```python
from build123d import *

# Parameters (mm, degrees)
SKETCH_1_R          = 16.5
EXTRUDE_1_DEPTH     = 22.7
SKETCH_2_R          = 18.5
EXTRUDE_2_DEPTH     = 19
SKETCH_3_R          = 1.5
CUT_EXTRUDE_1_DEPTH = 2
SKETCH_4_R          = 5.5
EXTRUDE_3_DEPTH     = 6
SKETCH_5_R          = 3
EXTRUDE_4_DEPTH     = 15.5
SKETCH_6_R          = 5
EXTRUDE_5_DEPTH     = 2.8
SKETCH_7_W          = 3.619294394
SKETCH_7_H          = 1.78180647
EXTRUDE_6_DEPTH     = 3.5


with BuildPart() as part:
    # 草图1 → 凸台-拉伸1 (new body)
    with BuildSketch(Plane.XY):
        Circle(SKETCH_1_R)
    extrude(amount=EXTRUDE_1_DEPTH)

    # 草图2 → 凸台-拉伸2 (add)
    with BuildSketch(Plane.XY.offset(22.7)):
        Circle(SKETCH_2_R)
    extrude(amount=EXTRUDE_2_DEPTH)

    # 草图3 → 切除-拉伸1 (cut)
    with BuildSketch(Plane.XY.offset(41.7)):
        with Locations((15.5, 0)):
            Circle(SKETCH_3_R)
        with Locations((7.75, -13.423393759)):
            Circle(SKETCH_3_R)
        with Locations((-7.75, -13.423393759)):
            Circle(SKETCH_3_R)
        with Locations((-15.5, 0)):
            Circle(SKETCH_3_R)
        with Locations((-7.75, 13.423393759)):
            Circle(SKETCH_3_R)
        with Locations((7.75, 13.423393759)):
            Circle(SKETCH_3_R)
    extrude(amount=-CUT_EXTRUDE_1_DEPTH, mode=Mode.SUBTRACT)

    # 草图4 → 凸台-拉伸3 (add)
    with BuildSketch(Plane.XY.offset(41.7)):
        with Locations((0, 7)):
            Circle(SKETCH_4_R)
    extrude(amount=EXTRUDE_3_DEPTH)

    # 草图5 → 凸台-拉伸4 (add)
    with BuildSketch(Plane.XY.offset(47.7)):
        with Locations((0, 7)):
            Circle(SKETCH_5_R)
    extrude(amount=EXTRUDE_4_DEPTH)

    # 草图6 → 凸台-拉伸5 (add)
    with BuildSketch(Plane(origin=(0, 0, 0), x_dir=(-1, 0, 0), z_dir=(0, 0, -1))):
        Circle(SKETCH_6_R)
    extrude(amount=EXTRUDE_5_DEPTH)

    # 草图7 → 凸台-拉伸6 (add)
    with BuildSketch(Plane(origin=(0, 0, 0), x_dir=(-1, 0, 0), z_dir=(0, 0, -1))):
        with Locations((0, 11.99935295)):
            Rectangle(SKETCH_7_W, SKETCH_7_H)
        with Locations((0, -11.99935295)):
            Rectangle(SKETCH_7_W, SKETCH_7_H)
    extrude(amount=EXTRUDE_6_DEPTH)


solid = part.part
```
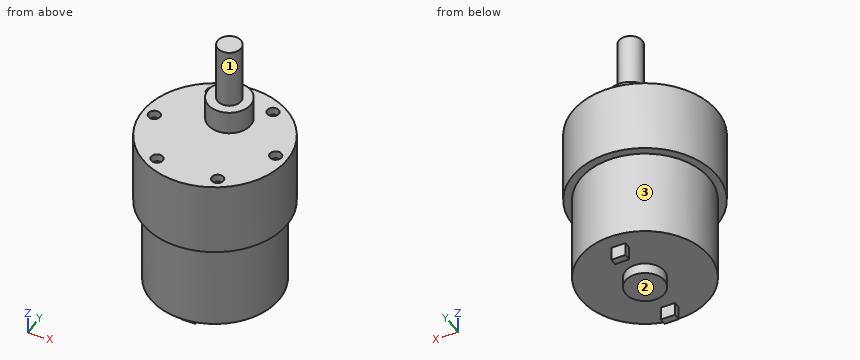
The model under review builds one solid part; all positions refer to its coordinate system, in mm. Face numbers are marked on the shaded views. A direction names the side the tool comes from. Round coordinates to 2 decimals unless told otherwise and drop trailing zeros. Order: outer loops, then holes, each group sorted by start corner. A loop starts at its lowest first (then second) coordinate and runs counter-clockwise, first axis right, second up. Notation, with made-up numbers: (40, -18.75) -> (87, -18.75) arc R13 ccw to (87, -3.75) -> close; hole circle Ø4 at (-9.5, 35.5). An arc over 180 degrees is marked (long way). Use a Markdown table: item, result.
Q1. For line 1 (Y direction, x = 7.75, z = 40.25); line 2 (Z direction, x = 13.5, y = 11); line 3 (Z direction, x = 15, y = 2.5), list the stretches that pass through material, from the lowest coordinate up.
Values:
| item | result |
|---|---|
| line 1 | y = -16.8 to -14.92, -11.92 to 11.92, 14.92 to 16.8 |
| line 2 | z = 22.7 to 41.7 |
| line 3 | z = 0 to 41.7 |
Q2. We need section B-B on x = 0. Write out the cut boundary in (y, z).
Values:
| item | result |
|---|---|
| outline | (-18.5, 22.7) -> (-16.5, 22.7) -> (-16.5, 0) -> (-12.89, 0) -> (-12.89, -3.5) -> (-11.11, -3.5) -> (-11.11, 0) -> (-5, 0) -> (-5, -2.8) -> (5, -2.8) -> (5, 0) -> (11.11, 0) -> (11.11, -3.5) -> (12.89, -3.5) -> (12.89, 0) -> (16.5, 0) -> (16.5, 22.7) -> (18.5, 22.7) -> (18.5, 41.7) -> (12.5, 41.7) -> (12.5, 47.7) -> (10, 47.7) -> (10, 63.2) -> (4, 63.2) -> (4, 47.7) -> (1.5, 47.7) -> (1.5, 41.7) -> (-18.5, 41.7) -> close |
Q3. Tool access review of the marked faces 1, 2 and 3: name each direction out of +Z, -Z, +X, -X, +Y, -Y from which nothing blocks a thin tool from reaching the whole face with its end or side.
Values:
| item | result |
|---|---|
| face 1 | +Z |
| face 2 | -Z, +X, -X |
| face 3 | -Z |
Q4. Clearance check with flat-ended pins moving along their axes: P1, Ø1.4, axis at y = -12, z = -1.5, coming from the -X side; P2, Ø6, axis at x = 0, y = 14, coming from the +Z side; P3, Ø2.5, axis at x = -15.5, y = -0.5, coming from the +Z side. State where each tip first meets the part, or that it passes through.
Values:
| item | result |
|---|---|
| P1 | stops at x = -1.81 |
| P2 | stops at z = 47.7 |
| P3 | stops at z = 41.7 |
Q5. We need section A-A on y = 0. Write out the cut boundary in (x, z), then the cut area to 3 significant figures.
Values:
| item | result |
|---|---|
| outline | (-18.5, 22.7) -> (-16.5, 22.7) -> (-16.5, 0) -> (-5, 0) -> (-5, -2.8) -> (5, -2.8) -> (5, 0) -> (16.5, 0) -> (16.5, 22.7) -> (18.5, 22.7) -> (18.5, 41.7) -> (17, 41.7) -> (17, 39.7) -> (14, 39.7) -> (14, 41.7) -> (-14, 41.7) -> (-14, 39.7) -> (-17, 39.7) -> (-17, 41.7) -> (-18.5, 41.7) -> close |
| area | 1,470 mm^2 |
Q6. We need section D-D on x = 7.75. Write out the cut boundary in (y, z).
Values:
| item | result |
|---|---|
| outline | (-16.8, 22.7) -> (-14.57, 22.7) -> (-14.57, 0) -> (14.57, 0) -> (14.57, 22.7) -> (16.8, 22.7) -> (16.8, 41.7) -> (14.92, 41.7) -> (14.92, 39.7) -> (11.92, 39.7) -> (11.92, 41.7) -> (-11.92, 41.7) -> (-11.92, 39.7) -> (-14.92, 39.7) -> (-14.92, 41.7) -> (-16.8, 41.7) -> close |
Q7. We need section C-C on z = 8. Write out the cut boundary in (x, y), then the cut area to 3 significant figures.
Values:
| item | result |
|---|---|
| outline | circle Ø33 at (0, 0) |
| area | 855 mm^2 |
